Autodesk Inventor part; units mm, degrees
ref_plane "YZ Plane" through (0, 0, 0) normal (1, 0, 0) x (0, 1, 0)
ref_plane "XZ Plane" through (0, 0, 0) normal (0, 1, 0) x (-1, 0, 0)
ref_plane "XY Plane" through (0, 0, 0) normal (0, 0, 1) x (1, 0, 0)
sketch "Absorber-Base" plane through (0, 0, 0) normal (0, 0, 1) x (1, 0, 0)
  line L0 (-10, 10) -> (10, 10)
  line L1 (10, 10) -> (10, -10)
  line L2 (10, -10) -> (-10, -10)
  line L3 (-10, -10) -> (-10, 10)
  line L4 (-10, 10) -> (10, -10) construction
  line L5 (10, 10) -> (-10, -10) construction
  point P0 (0, 0)
  dimension "d0" = 20
extrude "Gesamtvolumen" add sketch "Absorber-Base" along normal blind 55
sketch "Skizze2" plane through (0, 0, 0) normal (0, 1, 0) x (-1, 0, 0)
  line L0 (-12.9394, 0) -> (12.9394, 0)
  line L1 (10, 0) -> (10, 55)
  line L2 (-10, 0) -> (-10, 55)
  line L3 (10, 0) -> (-10, 0)
  line L4 (-10, 0) -> (-10, 10)
  line L5 (-10, 10) -> (10, 10)
  line L6 (10, 10) -> (10, 0)
  line L7 (-10, 55) -> (10, 55)
  line L8 (0, 55) -> (10, 10)
  line L9 (0, 55) -> (-10, 10)
  point P0 (0, 0)
  point P1 (10, 10)
  dimension "d6" = 10
extrude "Cutaway" cut sketch "Skizze2" along normal mid plane 20 contours L2 L7 L9 | L8 L7 L1
pattern_circular "Runde Anordnung1" count 2 over 90 about axis through (0, 0, -10) along (0, 0, 1) of "Cutaway"
equation "\"d0\" = Base_Seitenlänge"
equation "\"d1\" = Gesamthöhe"
equation "\"d6\" = Base_Höhe"
equation "\"d7\" = Base_Seitenlänge"
equation "\"Base_Seitenlänge\" = 20"
equation "\"Base_Höhe\" = 10"
equation "\"Gesamthöhe\" = 55"
properties part number "Absorber - IHF-Mini"
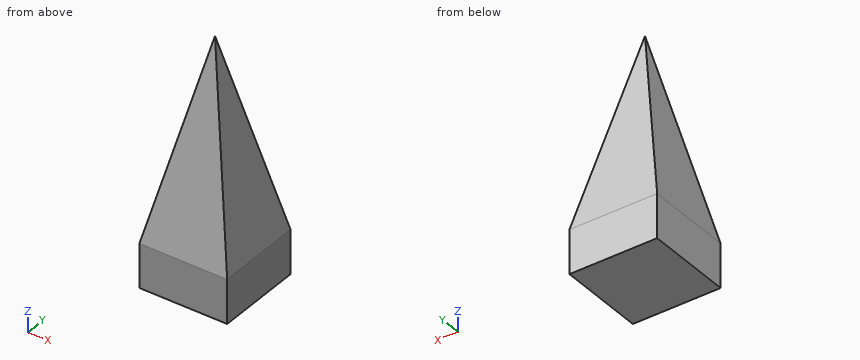
The model under review builds one solid part; all positions refer to its coordinate system, in mm. Round coordinates to 2 decimals unless told otherwise and drop trailing zeros. Loops run counter-clockwise (first coordinate to the right, second up) from the corner with the lowest first, then second, coordinate; pieces in that order, holes last. Notation, with made-up numbers: (55.25, -27.5) -> (80.25, -27.5) arc R15 ccw to (80.25, -8.5) -> close; hole circle Ø8 at (48, 30.25). An arc over 180 degrees is marked (long way). One line per question, with ' | ' between items. Start each with the question number.
Item 1: Add section A-A, the plane x = -5.5. Write out the cut boundary in (y, z).
Item 2: Add section B-B, the plane y = 3.5. Write out the cut boundary in (x, z), then the cut area to 3 significant figures.
Item 3: Wall thickness on line 1 along Y through (x, z) = (-0.25, 24); line 2 along Y through (x, z) = (4.5, 21.5); line 3 along X through (y, z) = (2, 28): over which ranges is each line inside the solid? List them lowest first. Write a range as [from, to].
Item 4: For pin 1 (6 mm diameter, centred on x = 3, z = 28.5, fed in from -Y); pin 2 (1.5 mm diameter, centred on x = -2, z = 30, fed in from -Y); pin 3 (2 mm diameter, centred on y = -5, z = 18.5, fed in from +X), all flat-tipped, find the tip position at first contact; note any pin that passes through.
Item 5: Add section C-C, the plane z = 23.5. Write out the cut boundary in (x, y).
Item 6: Add section D-D, the plane z = 47.5. Write out the cut boundary in (x, y).
Return value:
1) outline: (-10, 0) -> (10, 0) -> (10, 10) -> (5.5, 30.25) -> (-5.5, 30.25) -> (-10, 10) -> close
2) outline: (-10, 0) -> (10, 0) -> (10, 10) -> (3.5, 39.25) -> (-3.5, 39.25) -> (-10, 10) -> close | area: 595 mm2
3) line 1: y = [-6.89, 6.89] | line 2: y = [-7.44, 7.44] | line 3: x = [-6, 6]
4) pin 1: stops at y = -6.56 | pin 2: stops at y = -5.72 | pin 3: stops at x = 8.33
5) outline: (-7, -7) -> (7, -7) -> (7, 7) -> (-7, 7) -> close
6) outline: (-1.67, -1.67) -> (1.67, -1.67) -> (1.67, 1.67) -> (-1.67, 1.67) -> close
